```python
from build123d import *

# Parameters (mm, degrees)
CYLINDER_R     = 0.5
CYLINDER_DEPTH = 0.3
BOX003_W       = 45.9
BOX003_H       = 74
BOX003_DEPTH   = 0.3


with BuildPart() as cylinder:
    # Cylinder → Cylinder (new body)
    with BuildSketch(Plane(origin=(1, 6.5, 11.9), x_dir=(1, 0, 0), z_dir=(0, 0, 1))):
        Circle(CYLINDER_R)
    extrude(amount=CYLINDER_DEPTH)


with BuildPart() as displayframe001:
    # Box003 → Box003 (new body)
    with BuildSketch(Plane(origin=(1, -67.5, 11.9), x_dir=(1, 0, 0), z_dir=(0, 0, 1))):
        with Locations((22.95, 37)):
            Rectangle(BOX003_W, BOX003_H)
    extrude(amount=BOX003_DEPTH)

    # Fusion: union Cylinder
    add(cylinder.part)


solid = displayframe001.part
```
Input: part model. Units: mm. Frame: model coordinates. Coordinates: 2 decimals unless noted, no trailing zeros. Loops run counter-clockwise (first coordinate to the right, second up) from the corner with the lowest first, then second, coordinate; pieces in that order, holes last. Notation, with made-up numbers: (68, -39) - (84, -39) arc R16 cw to (84, -17) - close; hole circle Ø3 at (28.25, 66.25). An arc over 180 degrees is marked (long way). Answer in a Markdown table with one row per item.
(1) Cut plane A-A on z = 12.15. Output: boundary loops of the cut face in (x, y).
Model answer:
| item | result |
|---|---|
| outline | (1, -67.5) - (46.9, -67.5) - (46.9, 6.5) - (1.5, 6.5) arc R0.5 ccw (long way) to (1, 6) - close |
(2) Mould query, pull axis Z, two halves, no side actions, for faces 1 (the face through (23, -30, 11.9)), 2 (the face through (23, -30, 12.2)). Classes: pulls with the +Z half, pulls with the -Z half, needs draft (parallel to the pull), parting line crosses it, or undercut.
Model answer:
| item | result |
|---|---|
| face 1 | pulls with the -Z half |
| face 2 | pulls with the +Z half |
(3) Material intervals for L1, parallel to Y at x = 4.5, z = 12; L2, parallel to X at y = -26.5, z = 12.15, sorted ascending. Write a range as from..to.
Model answer:
| item | result |
|---|---|
| L1 | y = -67.5..6.5 |
| L2 | x = 1..46.9 |
